Answer from the drawing. Dimensions are ordinates in mm from the lowest x, y and z of the part. A direction names the side the tool comes from. Give positions to 0.01 mm unless a question says otherwise; leave off trailing zeros. Loops run counter-clockwise (first coordinate to the right, second up) from the corner with the lowest first, then second, coordinate; pieces in that order, holes last.
Item 1: Section D-D, the plane z = 13 is taken. Give the vertices of the cut face in (x, y), and give its area (3 significant figures).
Item 2: Each of these flat-tipped pins is pushed along its axis until it touches: pin 1 Ø2 at (x, z) = (16.5, 7) entering from +Y; pin 2 Ø6 at (y, z) = (20, 13.5) entering from +X (1 decimal); pin 3 Ø6 at (y, z) = (4.5, 5.5) entering from -X; pin 4 Ø1 at (x, z) = (12.5, 10.5) entering from -Y. Where does it stop, or does it pass through?
Item 3: A tool of negligible diameter and unlimited length cuts with its end or side. For the marked faces 1, 2 and 3, from which of +Z, -Z, +X, -X, +Y, -Y can it reach the whole face along a straight path? Write none if from no direction.
Item 4: Section C-C, the plane z = 8.25 is taken. Give the vertices of the cut face in (x, y) (1 decimal).
Item 5: The mould has two halves that part along X. Classify the marked faces 4, 5 and 6: pulls with the +X half, pulls with the -X half, needs draft (parallel to the pull), parting line crosses it, or undercut.
Item 6: Consider line 1 along X through (y, z) = (13.25, 8.75) (1 decimal); line 2 along Z through (x, y) = (11.25, 13.5); line 3 along Y through (x, z) = (5, 5.5). Determine where each line is inside the solid, lowest interval first.
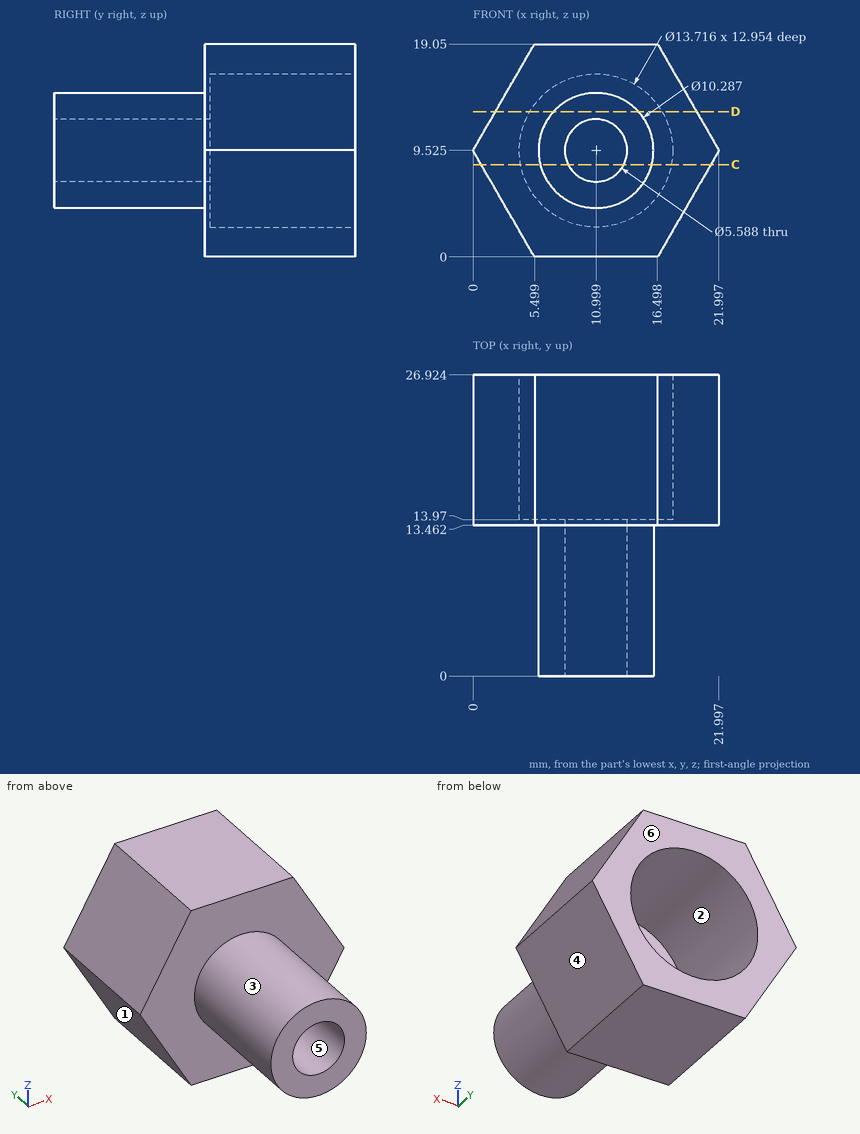
Worked answers:
1. outline: (2.01, 13.46) - (7.21, 13.46) - (7.21, 0) - (14.79, 0) - (14.79, 13.46) - (19.99, 13.46) - (19.99, 26.92) - (16.91, 26.92) - (16.91, 13.97) - (5.09, 13.97) - (5.09, 26.92) - (2.01, 26.92) - close
1. area: 191 mm2
2. pin 1: stops at y = 26.92
2. pin 2: stops at x = 21.4
2. pin 3: stops at x = 5.96
2. pin 4: passes through
3. face 1: -Z, -X, +Y, -Y
3. face 2: +Y
3. face 3: -Y
4. outline: (0.7, 13.5) - (6, 13.5) - (6, 0) - (8.5, 0) - (8.5, 14) - (4.3, 14) - (4.3, 26.9) - (0.7, 26.9) - close; (13.5, 0) - (16, 0) - (16, 13.5) - (21.3, 13.5) - (21.3, 26.9) - (17.7, 26.9) - (17.7, 14) - (13.5, 14) - close
5. face 4: pulls with the +X half
5. face 5: undercut
5. face 6: needs draft
6. line 1: x = 5.9 to 8.3, 13.7 to 16.1
6. line 2: z = 0 to 6.74, 12.31 to 19.05
6. line 3: y = 13.46 to 26.92
